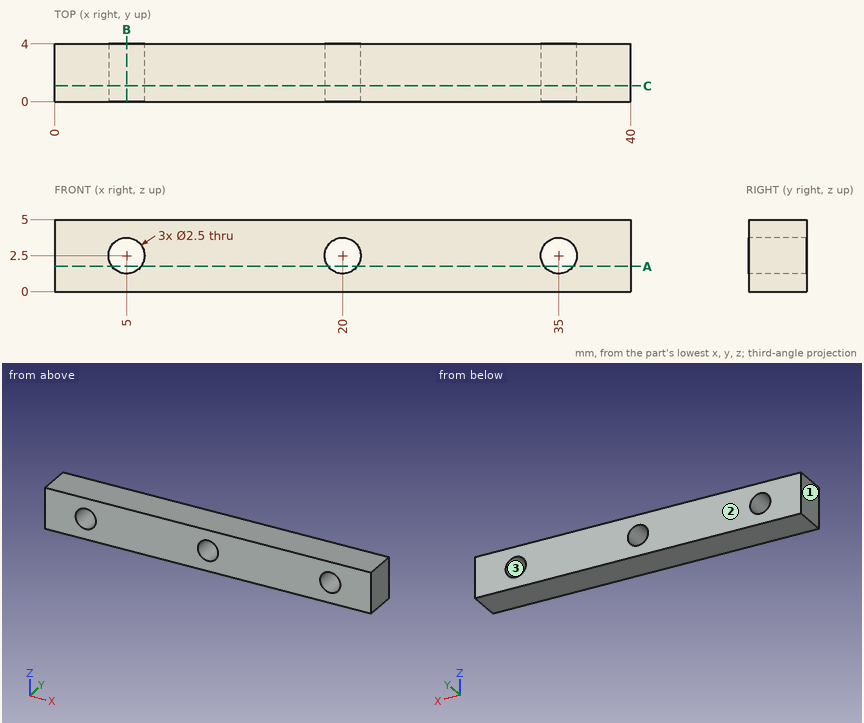
Geometry check sheet. Reference: drawing and pictorial views, mm from the part's lowest x, y, z. Coordinates: 2 decimals unless noted, no trailing zeros. Write each loop counter-clockwise with the first axis right and the second up, starting at its lowest first coordinate (ties: lowest second). Pieces come first, ordered by that corner, then holes.
Item 1: Depth check by flat-ended pin: pin 1 Ø1 at (x, z) = (13, 3.5) entering from -Y. Enter the tip coordinate at first touch or a pass-through.
Numbers:
pin 1: stops at y = 0
Item 2: Scan lines: probe 1 along X at (y, z) = (2.95, 2.5); probe 2 along Z at (x, y) = (35, 2.35); probe 3 along X at (y, z) = (1.2, 1.9). Record each from-to range of solid material in increasing order.
Numbers:
probe 1: x = 0 to 3.75, 6.25 to 18.75, 21.25 to 33.75, 36.25 to 40
probe 2: z = 0 to 1.25, 3.75 to 5
probe 3: x = 0 to 3.9, 6.1 to 18.9, 21.1 to 33.9, 36.1 to 40
Item 3: Mould release check, pull along X, two halves, no side actions. Record for the marked faces 1, 2 and 3: released by +X, released by -X, zero draft, split by the parting line, or undercut.
Numbers:
face 1: released by -X
face 2: zero draft
face 3: undercut
Item 4: Cross-section at A-A on z = 1.75. Record the boundary of the cut face in (x, y).
Numbers:
outline: (0, 0) - (4, 0) - (4, 4) - (0, 4) - close; (6, 0) - (19, 0) - (19, 4) - (6, 4) - close; (21, 0) - (34, 0) - (34, 4) - (21, 4) - close; (36, 0) - (40, 0) - (40, 4) - (36, 4) - close
Item 5: Cross-section at B-B on x = 5. Record the boundary of the cut face in (y, z).
Numbers:
outline: (0, 0) - (4, 0) - (4, 1.25) - (0, 1.25) - close; (0, 3.75) - (4, 3.75) - (4, 5) - (0, 5) - close
Item 6: Cross-section at C-C on y = 1.1. Record the boundary of the cut face in (x, z).
Numbers:
outline: (0, 0) - (40, 0) - (40, 5) - (0, 5) - close; hole circle Ø2.5 at (5, 2.5); hole circle Ø2.5 at (20, 2.5); hole circle Ø2.5 at (35, 2.5)
